Geometry check sheet. Reference: drawing and pictorial views, mm from the part's lowest x, y, z. A direction names the side the tool comes from. Coordinates: 2 decimals unless noted, no trailing zeros. Write each loop counter-clockwise with the first axis right and the second up, starting at its lowest first coordinate (ties: lowest second). Pieces come first, ordered by that corner, then holes. Notation, with made-up numbers: (0.5, -31.5) -> (38.5, -31.5) arc R35 cw to (38.5, 3.5) -> close; hole circle Ø1 at (74.25, 85). An arc over 180 degrees is marked (long way). Use a Markdown table: item, result. Add a question column.
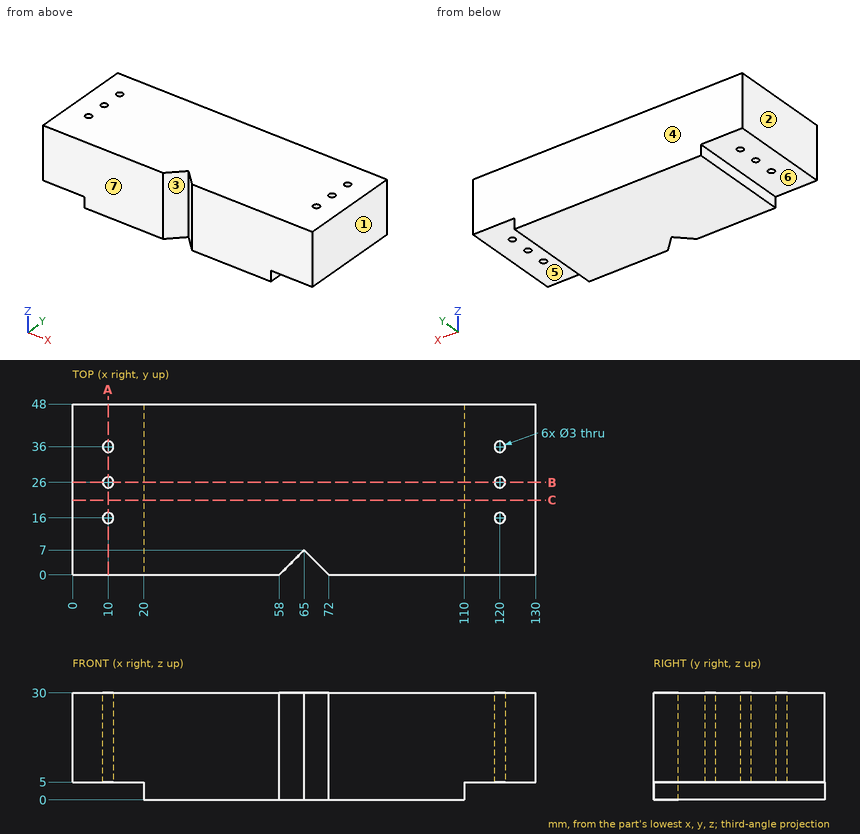
1) Cross-section at B-B on y = 26. Record the boundary of the cut face in (x, z).
2) Cross-section at C-C on y = 21. Record the boundary of the cut face in (x, z), then the cut area to 3 significant figures.
3) Thickness scan on L1, parallel to Y at x = 120, z = 21.5; L2, parallel to Z at x = 117, y = 28; L3, parallel to X at y = 28, z = 4. Record the ranges inside material, lowest first.
4) Cross-section at A-A on x = 10. Record the boundary of the cut face in (y, z).
5) Release check for a two-part mould opening along X. For the marked faces 1, 2, 3 and 4 record: released by +X, released by -X, zero draft, split by the parting line, or undercut.
6) Set-up check for the marked faces 5, 6 and 7: record each of +Z, -Z, +X, -X, +Y, -Y from which the full face is reachable in a straight line by a thin tool's end or side.
7) Gauge pin test, flat ends, axial feed: pin 1 (5 mm diameter, centred on x = 120, y = 36, fed in from -Z); pin 2 (1.5 mm diameter, centred on y = 13.5, z = 3, fed in from +X); pin 3 (5.5 mm diameter, centred on y = 22, z = 2, fed in from -X). Record the tip position at first contact, or that the pin passes through.
Returned:
| question | item | result |
|---|---|---|
| 1 | outline | (0, 5) -> (8.5, 5) -> (8.5, 30) -> (0, 30) -> close; (11.5, 5) -> (20, 5) -> (20, 0) -> (110, 0) -> (110, 5) -> (118.5, 5) -> (118.5, 30) -> (11.5, 30) -> close; (121.5, 5) -> (130, 5) -> (130, 30) -> (121.5, 30) -> close |
| 2 | outline | (0, 5) -> (20, 5) -> (20, 0) -> (110, 0) -> (110, 5) -> (130, 5) -> (130, 30) -> (0, 30) -> close |
| 2 | area | 3,700 mm² |
| 3 | L1 | y = 0 to 14.5, 17.5 to 24.5, 27.5 to 34.5, 37.5 to 48 |
| 3 | L2 | z = 5 to 30 |
| 3 | L3 | x = 20 to 110 |
| 4 | outline | (0, 5) -> (14.5, 5) -> (14.5, 30) -> (0, 30) -> close; (17.5, 5) -> (24.5, 5) -> (24.5, 30) -> (17.5, 30) -> close; (27.5, 5) -> (34.5, 5) -> (34.5, 30) -> (27.5, 30) -> close; (37.5, 5) -> (48, 5) -> (48, 30) -> (37.5, 30) -> close |
| 5 | face 1 | released by +X |
| 5 | face 2 | released by -X |
| 5 | face 3 | undercut |
| 5 | face 4 | zero draft |
| 6 | face 5 | -Z, +X, +Y, -Y |
| 6 | face 6 | -Z, -X, +Y, -Y |
| 6 | face 7 | +Z, -Z, +X, -X, -Y |
| 7 | pin 1 | stops at z = 5 |
| 7 | pin 2 | stops at x = 110 |
| 7 | pin 3 | stops at x = 20 |
